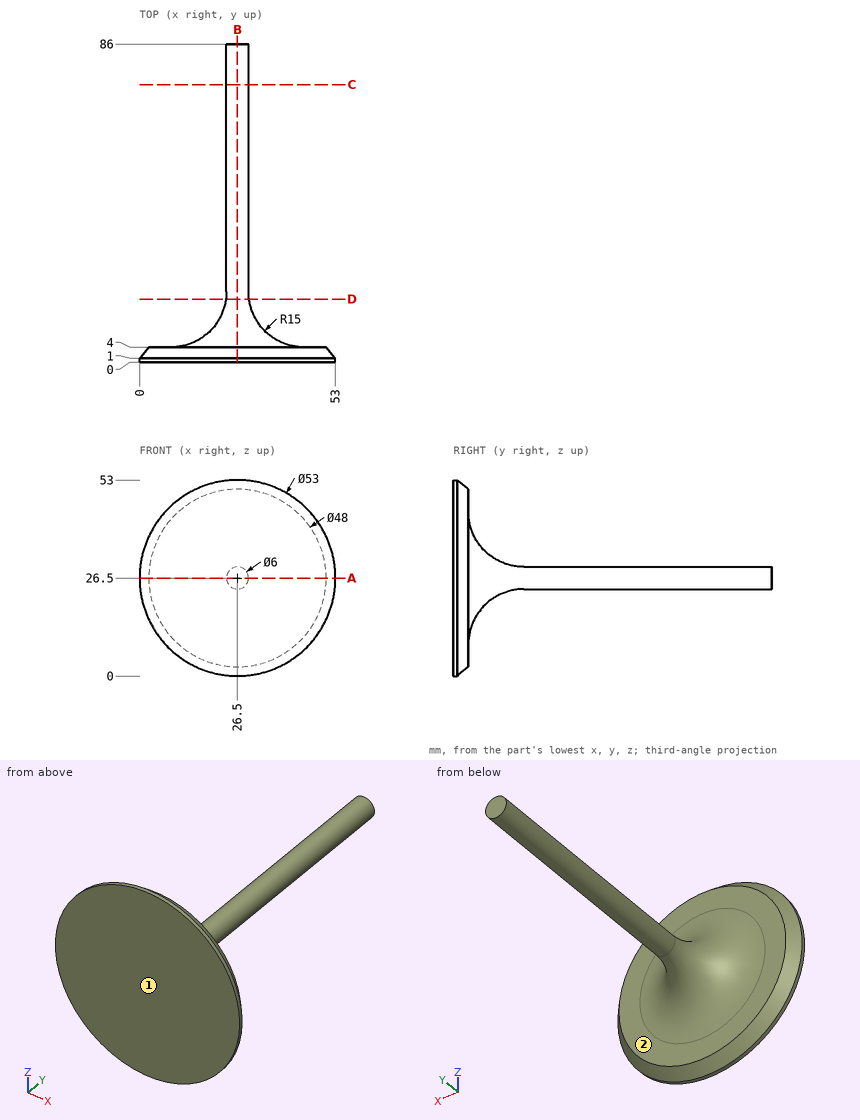
The figure shows three views and two pictorial views of one solid part (mm, origin at its lowest corner). Answer the questions. A direction names the side the tool comes from. Coordinates: 2 decimals unless noted, no trailing zeros. Order: outer loops, then holes, each group sorted by start corner. A loop starts at its lowest first (then second) coordinate and runs counter-clockwise, first axis right, second up.
Q1. A cutting plane is placed at B-B, the plane x = 26.5. Write down the section's boundary in (y, z).
Q2. A cutting plane is placed at A-A, the plane z = 26.5. Write down the section's boundary in (x, y).
Q3. Given P1, Ø12, axis at x = 14, y = 25.5, coming from the +Z side; P2, Ø5, axis at y = 23, z = 24.5, coming from the -X side; P3, Ø6, axis at x = 47.5, z = 32, coming from the +Y side, each flat-ended and moving along its own axis, determine where each tip first touches the part or whether it passes through.
Q4. A cutting plane is placed at C-C, the plane y = 75. Write down the section's boundary in (x, z).
Q5. Which of the six approach directions +Z, -Z, +X, -X, +Y, -Y give full straight-line access (tool end or side, diameter ignored) to the marked faces 1 and 2?
Q6. Consider line 1 (Y direction, x = 28, z = 4.5); line 2 (Y direction, x = 36, z = 49); line 3 (X direction, y = 72, z = 27). Determine where each line is inside the solid, lowest interval first.
Q7. A cutting plane is placed at D-D, the plane y = 17. Write down the section's boundary in (x, z).
Answers follow:
1. outline: (0, 0) - (1, 0) - (4, 2.5) - (4, 8.5) arc R15 cw to (19, 23.5) - (86, 23.5) - (86, 29.5) - (19, 29.5) arc R15 cw to (4, 44.5) - (4, 50.5) - (1, 53) - (0, 53) - close
2. outline: (0, 0) - (53, 0) - (53, 1) - (50.5, 4) - (44.5, 4) arc R15 cw to (29.5, 19) - (29.5, 86) - (23.5, 86) - (23.5, 19) arc R15 cw to (8.5, 4) - (2.5, 4) - (0, 1) - close
3. P1: passes through
3. P2: stops at x = 23.5
3. P3: stops at y = 4
4. outline: circle Ø6 at (26.5, 26.5)
5. face 1: +Z, -Z, +X, -X, -Y
5. face 2: +Y
6. line 1: y = 0 to 4
6. line 2: y = 0 to 3.49
6. line 3: x = 23.54 to 29.46
7. outline: circle Ø6.27 at (26.5, 26.5)
